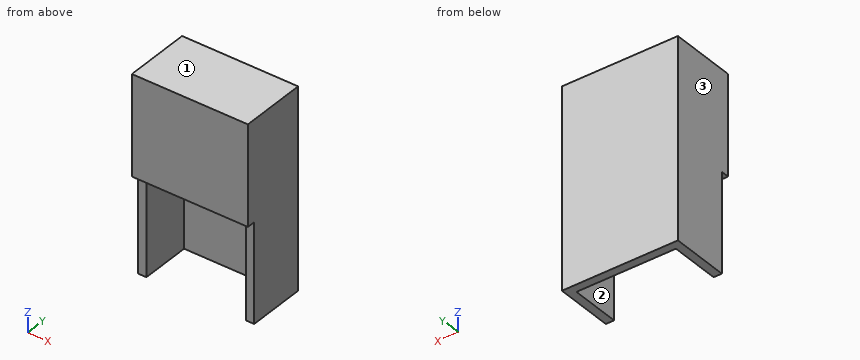
```python
from build123d import *

# Parameters (mm, degrees)
F0_W     = 70
F0_H     = 120
F1_DEPTH = 40
F2_W     = 60
F2_H     = 30
F3_DEPTH = 60
F4_W     = 70
F4_H     = 59.779245
F5_DEPTH = 5


with BuildPart() as f1:
    # F0 (on Front) → F1 (new body)
    with BuildSketch(Plane.XZ):
        with Locations((7.426471, 60)):
            Rectangle(F0_W, F0_H)
    extrude(amount=F1_DEPTH)

    # F2 (on Top) → F3 (cut)
    with BuildSketch(Plane.XY):
        with Locations((7.426471, -20)):
            Rectangle(F2_W, F2_H)
    extrude(amount=F3_DEPTH, mode=Mode.SUBTRACT)

    # F4 (on face) → F5 (cut)
    with BuildSketch(Plane.XZ.offset(40)):
        with Locations((7.426471, 29.889622)):
            Rectangle(F4_W, F4_H)
    extrude(amount=-F5_DEPTH, mode=Mode.SUBTRACT)


solid = f1.part
```
Geometry: final body of the model. Coordinates: model frame, mm. Face numbers are marked on the shaded views. Round coordinates to 2 decimals unless told otherwise and drop trailing zeros. Write each loop counter-clockwise with the first axis right and the second up, starting at its lowest first coordinate (ties: lowest second). Pieces come first, ordered by that corner, then holes.
Item 1: Section query C-C (y = -37). Return loops of the section in (x, z).
Item 2: Pin query (flat end, axial travel): P1, Ø5.5, axis at x = 40.5, z = 40, coming from the -Y side; P2, Ø15, axis at x = 9.5, y = -16, coming from the -Z side; P3, Ø5, axis at x = 19.5, z = 20, coming from the -Y side. Return the tip coordinate at first contact, or that it passes through.
Item 3: Mould query, pull axis X, two halves, no side actions, for the marked faces 1, 2 and 3. Classes: +X half, -X half, draft (parallel to the pull), parting line (faces both ways), or undercut.
Item 4: Section query A-A (y = -23.5). Return loops of the section in (x, z).
Item 5: Section query B-B (z = 33). Return loops of the section in (x, y).
Item 6: Material intervals for L1, parallel to Y at x = 5, z = 12; L2, parallel to Z at x = 33, y = -37.5; L3, parallel to Z at x = 5, y = -22, sorted ascending.
Completed:
1. outline: (-27.57, 59.78) - (42.43, 59.78) - (42.43, 120) - (-27.57, 120) - close
2. P1: stops at y = -35
2. P2: stops at z = 60
2. P3: stops at y = -5
3. face 1: draft
3. face 2: undercut
3. face 3: -X half
4. outline: (-27.57, 0) - (-22.57, 0) - (-22.57, 60) - (37.43, 60) - (37.43, 0) - (42.43, 0) - (42.43, 120) - (-27.57, 120) - close
5. outline: (-27.57, -35) - (-22.57, -35) - (-22.57, -5) - (37.43, -5) - (37.43, -35) - (42.43, -35) - (42.43, 0) - (-27.57, 0) - close
6. L1: y = -5 to 0
6. L2: z = 59.78 to 120
6. L3: z = 60 to 120
